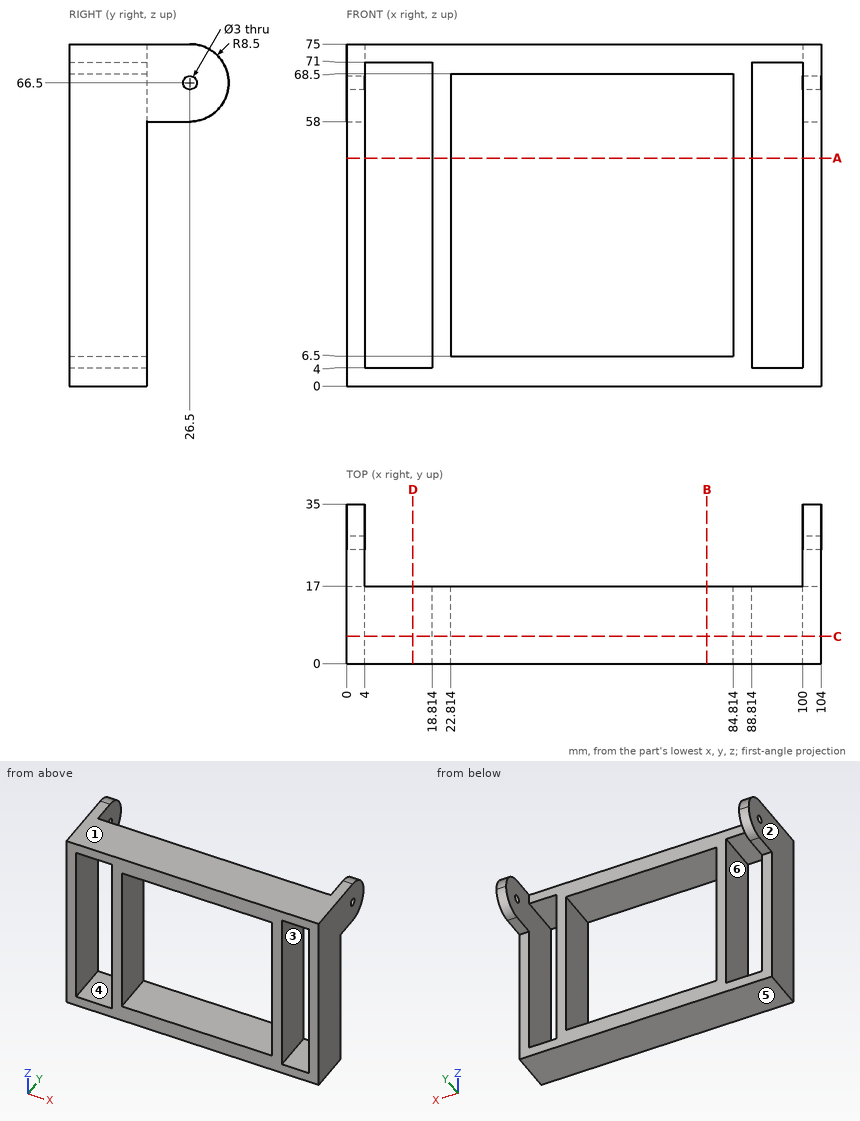
Source: three-view drawing plus pictorial views. Frame: mm from the lowest corner of the part. A direction names the side the tool comes from. Give positions to 0.01 mm unless a question says otherwise; leave off trailing zeros. Loops run counter-clockwise (first coordinate to the right, second up) from the corner with the lowest first, then second, coordinate; pieces in that order, holes last. Notation, with made-up numbers: M -31,0 L 25,0 A28 cw 25,26 Z; hole C 38.25,71 d5. An arc over 180 degrees is marked long. Put each result on its own line as item: value.
Q1. Line query: probe 1 along X at (y, z) = (13, 40); probe 2 along Z at (x, y) = (64, 9.5); probe 3 along X at (y, z) = (12, 6). Output: solid intervals per line, ascending. Write a range as [from, to].
Response values:
probe 1: x = [0, 4], [18.81, 22.81], [84.81, 88.81], [100, 104]
probe 2: z = [0, 6.5], [68.5, 75]
probe 3: x = [0, 4], [18.81, 88.81], [100, 104]
Q2. Reachability of the marked faces 5 and 6 from +Z, -Z, +X, -X, +Y, -Y: full face, straight path, thin tool, end or side. Return the list, or none.
Response values:
face 5: -Z, +X, -X, +Y, -Y
face 6: +Y, -Y
Q3. Section C-C (y = 6). Return the cut outline in (x, z), and give its area (3 significant figures).
Response values:
outline: M 0,0 L 104,0 L 104,75 L 0,75 Z; hole M 4,4 L 18.81,4 L 18.81,71 L 4,71 Z; hole M 22.81,6.5 L 84.81,6.5 L 84.81,68.5 L 22.81,68.5 Z; hole M 88.81,4 L 100,4 L 100,71 L 88.81,71 Z
area: 2,210 mm²
Q4. Pin query (flat end, axial travel): P1, Ø4.5, axis at x = 14.5, y = 6, coming from the -Z side; P2, Ø3, axis at x = 2, y = 20.5, coming from the -Z side. Return the tip coordinate at first contact, or that it passes through.
Response values:
P1: stops at z = 0
P2: stops at z = 58
Q5. Mould query, pull axis Z, two halves, no side actions, for the marked faces 1, 2, 3 and 4. Classes: released by +Z, released by -Z, zero draft, split by the parting line, or undercut.
Response values:
face 1: released by +Z
face 2: zero draft
face 3: undercut
face 4: undercut
Q6. Section A-A (z = 50). Return the cut outline in (x, y).
Response values:
outline: M 0,0 L 4,0 L 4,17 L 0,17 Z; M 18.81,0 L 22.81,0 L 22.81,17 L 18.81,17 Z; M 84.81,0 L 88.81,0 L 88.81,17 L 84.81,17 Z; M 100,0 L 104,0 L 104,17 L 100,17 Z
Q7. Section B-B (x = 79). Return the cut outline in (y, z).
Response values:
outline: M 0,0 L 17,0 L 17,6.5 L 0,6.5 Z; M 0,68.5 L 17,68.5 L 17,75 L 0,75 Z
Q8. Section D-D (x = 14.5). Return the cut outline in (y, z), and give its area (3 significant figures).
Response values:
outline: M 0,0 L 17,0 L 17,4 L 0,4 Z; M 0,71 L 17,71 L 17,75 L 0,75 Z
area: 136 mm²
